Here's how the part is built. I have some questions about the finished solid (model axes, mm). A direction names the side the tool comes from. Coordinates: 2 decimals unless noted, no trailing zeros. Loops run counter-clockwise (first coordinate to the right, second up) from the corner with the lowest first, then second, coordinate; pieces in that order, holes last. Notation, with made-up numbers: (21, -15) - (31, -15) arc R19 ccw to (31, 1) - close; hole circle Ø1 at (21.5, -7). An arc over 180 degrees is marked (long way). Use a Markdown table: item, result.
Autodesk Inventor part; units mm, degrees
ref_plane "YZ Plane" through (0, 0, 0) normal (1, 0, 0) x (0, 1, 0)
ref_plane "XZ Plane" through (0, 0, 0) normal (0, 1, 0) x (-1, 0, 0)
ref_plane "XY Plane" through (0, 0, 0) normal (0, 0, 1) x (1, 0, 0)
sketch "Sketch1" plane through (0, 0, 0) normal (0, 1, 0) x (-1, 0, 0)
  line L0 (0, 0) -> (-13.27, 0)
  line L1 (-13.27, 0) -> (-13.27, 6.9)
  line L2 (-13.27, 6.9) -> (0, 6.9)
  line L3 (0, 6.9) -> (0, 0)
  line L4 (3, -3) -> (-16.27, -3)
  line L5 (-16.27, -3) -> (-16.27, 9.9)
  line L6 (-16.27, 9.9) -> (3, 9.9)
  line L7 (3, 9.9) -> (3, -3)
  point P0 (-6.635, -3)
  point P1 (-6.635, 0)
  point P2 (3, 3.45)
  dimension "d0" = 13.27
  dimension "d1" = 6.9
  dimension "d2" = 3
  dimension "d3" = 3
  dimension "d4" = 3
  dimension "d5" = 3
extrude "Extrusion1" add sketch "Sketch1" along normal blind 8.8
sketch "Sketch2" plane through (0, 0, 0) normal (0, -1, 0) x (1, 0, 0)
  line L0 (-3, 9.9) -> (16.27, 9.9)
  line L1 (16.27, -3) -> (-3, -3)
  line L2 (-3, 9.9) -> (16.27, 9.9)
  line L3 (16.27, 9.9) -> (16.27, -3)
  line L4 (16.27, -3) -> (-3, -3)
  line L5 (-3, -3) -> (-3, 9.9)
  point P0 (0, 0)
  point P1 (16.27, 9.9)
extrude "Extrusion2" add sketch "Sketch2" along normal blind 3
sketch "Sketch3" plane through (0, 0, 0) normal (0, 1, 0) x (1, 0, 0)
  line L0 (0, -6.9) -> (0, 0)
  line L1 (13.27, -6.9) -> (0, -6.9)
  line L2 (0, 0) -> (8.3, 0)
  line L3 (8.3, 0) -> (8.3, -6.9)
  line L4 (8.3, -6.9) -> (0, -6.9)
  line L5 (0, -6.9) -> (0, 0)
  dimension "d10" = 8.3
extrude "Extrusion3" cut sketch "Sketch3" against normal blind 3
equation "\"d3\" = d2"
equation "\"d5\" = d4"
properties part number "switch test v03"
Q1. Which directions (+Z, -Z, +X, -X, +Y, -Y) give clear straight access to the entire face, cutting with the end or side of a thin tool? Please do faces 1 (the face through (8.3, -1, 3)), 2 (the face through (7, 3, 0)), 3 (the face through (9, -3, 4)).
Check values:
| item | result |
|---|---|
| face 1 | +Y, -Y |
| face 2 | +Y |
| face 3 | +Z, -Z, +X, -X, -Y |
Q2. I want a section at D-D, the plane x = 11.5. Write out the boundary of the cut face in (y, z).
Check values:
| item | result |
|---|---|
| outline | (-3, -3) - (8.8, -3) - (8.8, 0) - (0, 0) - (0, 6.9) - (8.8, 6.9) - (8.8, 9.9) - (-3, 9.9) - close |
Q3. I want a section at B-B, the plane y = 7.25. Write out the boundary of the cut face in (x, z).
Check values:
| item | result |
|---|---|
| outline | (-3, -3) - (16.27, -3) - (16.27, 9.9) - (-3, 9.9) - close; hole (0, 0) - (13.27, 0) - (13.27, 6.9) - (0, 6.9) - close |
Q4. I want a section at A-A, the plane z = 3. Write out the boundary of the cut face in (x, y), then the cut area to 3 significant figures.
Check values:
| item | result |
|---|---|
| outline | (-3, -3) - (0, -3) - (0, 8.8) - (-3, 8.8) - close; (8.3, -3) - (16.27, -3) - (16.27, 8.8) - (13.27, 8.8) - (13.27, 0) - (8.3, 0) - close |
| area | 85.7 mm^2 |
Q5. If we mould it in two halves opening along Z, with no side actions, what happens to faces 4 (the face through (7, 3, 9.9)), 5 (the face through (0, 3, 3)), 6 (the face through (7, 3, -3)), 7 (the face through (7, 8.8, 8))? For each: pulls with the +Z half, pulls with the -Z half, needs draft (parallel to the pull), parting line crosses it, or undercut.
Check values:
| item | result |
|---|---|
| face 4 | pulls with the +Z half |
| face 5 | undercut |
| face 6 | pulls with the -Z half |
| face 7 | needs draft |
Q6. Please list where these lines run through material, in increasing order: L1, parallel to Z at x = 6, y = 0.5; L2, parallel to X at y = 6.75, z = 2.25; L3, parallel to X at y = -2.5, z = 5. Write a range as from..to.
Check values:
| item | result |
|---|---|
| L1 | -3..0, 6.9..9.9 |
| L2 | -3..0, 13.27..16.27 |
| L3 | -3..0, 8.3..16.27 |
Q7. I want a section at C-C, the plane x = 4.5. Write out the boundary of the cut face in (y, z).
Check values:
| item | result |
|---|---|
| outline | (-3, -3) - (8.8, -3) - (8.8, 0) - (-3, 0) - close; (-3, 6.9) - (8.8, 6.9) - (8.8, 9.9) - (-3, 9.9) - close |
Q8. Will these pins go through, and if not, where does the flat tip stop? P1, Ø1.5, axis at x = 10.5, z = 2, coming from the +Y side; P2, Ø2, axis at x = 5, z = 2, coming from the -Y side.
Check values:
| item | result |
|---|---|
| P1 | y = 0 |
| P2 | through |
